from build123d import *

# Parameters (mm, degrees)
EXTRUDE_1_DEPTH     = 19
SKETCH_3_R          = 27.5
CUT_EXTRUDE_1_DEPTH = 19
SKETCH_4_R          = 5.5
SKETCH_4_R_2        = 5.523267564
CUT_EXTRUDE_2_DEPTH = 30
SKETCH_5_R          = 27.5
SKETCH_5_R_2        = 24
EXTRUDE_2_DEPTH     = 2
SKETCH_6_W          = 12
SKETCH_6_H          = 6.6
CUT_EXTRUDE_3_DEPTH = 30
FILLET_1_R          = 1
FILLET_2_R          = 2


with BuildPart() as part:
    # 草图2 → 凸台-拉伸1 (new body)
    with BuildSketch(Plane.XY):
        Polygon((32, 10), (52, 10), (52, -10), (-52, -10), (-52, 10), (-32, 10), (-32, 57), (32, 57), align=None)
    extrude(amount=EXTRUDE_1_DEPTH)

    # 草图3 → 切除-拉伸1 (cut)
    with BuildSketch(Plane.XY.offset(19)):
        with Locations((0, 25)):
            Circle(SKETCH_3_R)
    extrude(amount=-CUT_EXTRUDE_1_DEPTH, mode=Mode.SUBTRACT)

    # 草图4 → 切除-拉伸2 (cut)
    with BuildSketch(Plane(origin=(0, 10, 0), x_dir=(1, 0, 0), z_dir=(0, 1, 0))):
        with Locations(Location((-42, -9.5, 0), (0, 0, 270))):
            Circle(SKETCH_4_R)
        with Locations(Location((42, -9.5, 0), (0, 0, 270))):
            Circle(SKETCH_4_R_2)
    extrude(amount=-CUT_EXTRUDE_2_DEPTH, mode=Mode.SUBTRACT)

    # 草图5 → 凸台-拉伸2 (add)
    with BuildSketch(Plane.XY.offset(19)):
        with Locations((0, 25)):
            Circle(SKETCH_5_R)
        with Locations((0, 25)):
            Circle(SKETCH_5_R_2, mode=Mode.SUBTRACT)
    extrude(amount=-EXTRUDE_2_DEPTH)

    # 草图6 → 切除-拉伸3 (cut)
    with BuildSketch(Plane(origin=(0, 0, 0), x_dir=(-1, 0, 0), z_dir=(0, 0, -1))):
        with Locations((0, -10)):
            Rectangle(SKETCH_6_W, SKETCH_6_H)
    extrude(amount=-CUT_EXTRUDE_3_DEPTH, mode=Mode.SUBTRACT)

    # 圆角1
    fillet_1_edges = [part.edges().sort_by_distance(p)[0] for p in [
        (-6, -6.7, 9.5),
        (6, -6.7, 9.5),
    ]]
    fillet(fillet_1_edges, radius=FILLET_1_R)

    # 圆角2
    fillet_2_edges = [part.edges().sort_by_distance(p)[0] for p in [
        (-32, 10, 9.5),
        (32, 10, 9.5),
    ]]
    fillet(fillet_2_edges, radius=FILLET_2_R)


solid = part.part
Input: part model. Units: mm. Frame: model coordinates. A direction names the side the tool comes from. Round coordinates to 2 decimals unless told otherwise and drop trailing zeros. Loops run counter-clockwise (first coordinate to the right, second up) from the corner with the lowest first, then second, coordinate; pieces in that order, holes last. Notation, with made-up numbers: (-20.5, -38) -> (26.5, -38) arc R15 ccw to (26.5, -25) -> close; hole circle Ø10 at (-32, 15). An arc over 180 degrees is marked (long way). Answer as a JSON object with one key per item and string values. Group by question number.
1) Section query C-C on y = 25. Output: boundary loops of the cut face in (x, z), plus the area to 3 significant figures.
2) Section query B-B on x = -42. Output: boundary loops of the cut face in (y, z).
3) Ray query, L1, parallel to Y at x = 0, z = 18.5; L2, parallel to X at y = 2, z = 9.5; L3, parallel to X at y = 2.25, z = 9.5. Return the intervals inside material, ascending.
4) Draft query along Y for faces 1 (the flat face through (6, -9, 9)), 2 (the cylindrical face through (-32.57, 10.6, 9.63)), 3 (the cylindrical face through (-17.69, 41.22, 18.01)). Return one class per face: +Y half, -Y half, draft (parallel to the pull), parting line (faces both ways), or undercut.
5) Reachability of faces 4 (the flat face through (-47, 10, 5)), 5 (the cylindrical face through (-20.269, 43.586, 8.619)), 6 (the flat face through (47, 10, 5)) from +Z, -Z, +X, -X, +Y, -Y: full face, straight path, thin tool, end or side. Return the list, or none.
6) Section query A-A on z = 9.5. Output: boundary loops of the cut face in (x, y).
7) Section query D-D on x = 42. Output: boundary loops of the cut face in (y, z).
8) Pin query (flat end, axial travel): pin 1 (5.5 mm diameter, centred on x = -46.5, z = 7, fed in from +Y); pin 2 (9.5 mm diameter, centred on y = 30.5, z = 5, fed in from +X). Return the tip coordinate at first contact, or that it passes through.
Reply:
{
 "1": {"outline": "(-32, 0) -> (-27.5, 0) -> (-27.5, 17) -> (-24, 17) -> (-24, 19) -> (-32, 19) -> close; (24, 17) -> (27.5, 17) -> (27.5, 0) -> (32, 0) -> (32, 19) -> (24, 19) -> close", "area": "185 mm2"},
 "2": {"outline": "(-10, 0) -> (10, 0) -> (10, 4) -> (-10, 4) -> close; (-10, 15) -> (10, 15) -> (10, 19) -> (-10, 19) -> close"},
 "3": {"L1": "y = -6.7 to 1, 49 to 57", "L2": "x = -52 to -47.5, -36.5 to -15.07, 15.07 to 36.48, 47.52 to 52", "L3": "x = -52 to -47.5, -36.5 to -15.45, 15.45 to 36.48, 47.52 to 52"},
 "4": {"face 1": "draft", "face 2": "+Y half", "face 3": "undercut"},
 "5": {"face 4": "+Z, -Z, -X, +Y", "face 5": "-Z", "face 6": "+Z, -Z, +X, +Y"},
 "6": {"outline": "(-52, -10) -> (-47.5, -10) -> (-47.5, 10) -> (-52, 10) -> close; (-36.5, -10) -> (-6, -10) -> (-6, -7.7) arc R1 cw to (-5, -6.7) -> (5, -6.7) arc R1 cw to (6, -7.7) -> (6, -10) -> (36.48, -10) -> (36.48, 10) -> (34, 10) arc R2 cw to (32, 12) -> (32, 57) -> (-32, 57) -> (-32, 12) arc R2 cw to (-34, 10) -> (-36.5, 10) -> close; (47.52, -10) -> (52, -10) -> (52, 10) -> (47.52, 10) -> close; hole circle Ø55 at (0, 25)"},
 "7": {"outline": "(-10, 0) -> (10, 0) -> (10, 3.98) -> (-10, 3.98) -> close; (-10, 15.02) -> (10, 15.02) -> (10, 19) -> (-10, 19) -> close"},
 "8": {"pin 1": "stops at y = 10", "pin 2": "stops at x = 32"}
}
